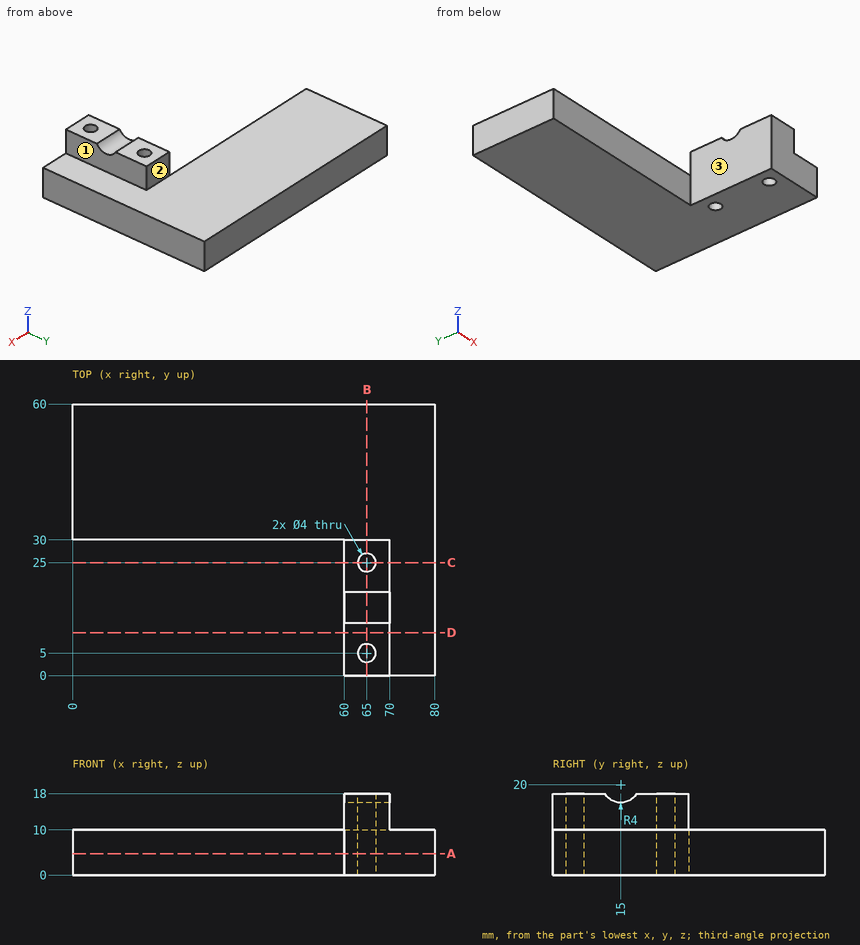
Design review of the part shown in the three views and the two pictorial views. Dimensions are in mm from the part's minimum x, y and z. A direction names the side the tool comes from. Give positions to 0.01 mm unless a question says otherwise; leave off trailing zeros. Loops run counter-clockwise (first coordinate to the right, second up) from the corner with the lowest first, then second, coordinate; pieces in that order, holes last. Notation, with made-up numbers: M 19,-25 L 76,-25 A20 cw 76,10 Z; hole C 60.5,-9.5 d10. An arc over 180 degrees is marked long. Put each result on its own line as item: value. Start each with the question number.
(1) Wall thickness on L1, parallel to X at y = 25, z = 12; L2, parallel to Y at x = 65, z = 17; L3, parallel to Y at x = 65, z = 5: over which ranges is each line inside the solid? List them lowest first.
(2) Add section A-A, the plane z = 4.75. Write out the cut boundary in (x, y).
(3) Add section D-D, the plane y = 9.5. Write out the cut boundary in (x, z), then the cut area to 3 significant figures.
(4) For pin 1 (3 mm diameter, centred on x = 65, y = 5, fed in from -Z); pin 2 (9 mm diameter, centred on y = 20, z = 15.5, fed in from +X); pin 3 (9 mm diameter, centred on x = 65, z = 15.5, fed in from +Y); pin 4 (3 mm diameter, centred on x = 20, z = 9, fed in from -Y), all flat-tipped, find the tip position at first contact; note any pin that passes through.
(5) Add section C-C, the plane y = 25. Write out the cut boundary in (x, z), then the cut area to 3 significant figures.
(6) Add section B-B, the plane x = 65. Write out the cut boundary in (y, z).
(7) Machinability: for the marked faces 1, 2 and 3, which of the approach directions +Z, -Z, +X, -X, +Y, -Y give a long, thin tool a straight path to every point of the face, cutting with its end or side? Answer none if there is none.
Result:
1. L1: x = 60 to 63, 67 to 70
1. L2: y = 0 to 3, 7 to 12.35, 17.65 to 23, 27 to 30
1. L3: y = 0 to 3, 7 to 23, 27 to 60
2. outline: M 0,30 L 60,30 L 60,0 L 80,0 L 80,60 L 0,60 Z; hole C 65,5 d4; hole C 65,25 d4
3. outline: M 60,0 L 80,0 L 80,10 L 70,10 L 70,18 L 60,18 Z
3. area: 280 mm^2
4. pin 1: passes through
4. pin 2: stops at x = 70
4. pin 3: stops at y = 30
4. pin 4: stops at y = 30
5. outline: M 60,0 L 63,0 L 63,18 L 60,18 Z; M 67,0 L 80,0 L 80,10 L 70,10 L 70,18 L 67,18 Z
5. area: 208 mm^2
6. outline: M 0,0 L 3,0 L 3,18 L 0,18 Z; M 7,0 L 23,0 L 23,18 L 18.46,18 A4 cw 11.54,18 L 7,18 Z; M 27,0 L 60,0 L 60,10 L 30,10 L 30,18 L 27,18 Z
7. face 1: +Z, +X, +Y, -Y
7. face 2: +Z, +X, -X, +Y
7. face 3: +Z, -Z, -X, -Y
